from build123d import *

# Parameters (mm, degrees)
F0_W     = 40
F0_H     = 52
F1_DEPTH = 20
F2_D     = 7.5
F3_W     = 20
F3_H     = 52
F4_DEPTH = 50
F5_W     = 20
F5_H     = 52
F6_DEPTH = 50


with BuildPart() as f1:
    # F0 (on Front) → F1 (new body)
    with BuildSketch(Plane.XZ):
        Rectangle(F0_W, F0_H)
    extrude(amount=F1_DEPTH)

    # F2 (through all)
    with Locations(Plane(origin=(0, 0, 0), x_dir=(1, 0, 0), z_dir=(0, 1, 0))):
        with Locations((12, 20), (-12, 20), (12, -20), (-12, -20)):
            Hole(F2_D / 2)

    # F3 (on face) → F4 (join)
    with BuildSketch(Plane(origin=(-20, 0, 0), x_dir=(0, -1, 0), z_dir=(-1, 0, 0))):
        with Locations((10, 0)):
            Rectangle(F3_W, F3_H)
    extrude(amount=F4_DEPTH)

    # F5 (on face) → F6 (join)
    with BuildSketch(Plane.YZ.offset(20)):
        with Locations((-10, 0)):
            Rectangle(F5_W, F5_H)
    extrude(amount=F6_DEPTH)


solid = f1.part
Model file for the job. Use its own axes, mm. Give positions to 0.01 mm unless a question says otherwise; leave off trailing zeros. Loops run counter-clockwise (first coordinate to the right, second up) from the corner with the lowest first, then second, coordinate; pieces in that order, holes last.
Item 1: Slice it at C-C (x = -12). Write the cut outline in (y, z).
Check values:
outline: (-20, -26) - (0, -26) - (0, -23.75) - (-20, -23.75) - close; (-20, -16.25) - (0, -16.25) - (0, 16.25) - (-20, 16.25) - close; (-20, 23.75) - (0, 23.75) - (0, 26) - (-20, 26) - close
Item 2: Slice it at B-B (z = 20). Write the cut outline in (x, y), plus the area to 3 significant figures.
Check values:
outline: (-70, -20) - (-15.75, -20) - (-15.75, 0) - (-70, 0) - close; (-8.25, -20) - (8.25, -20) - (8.25, 0) - (-8.25, 0) - close; (15.75, -20) - (70, -20) - (70, 0) - (15.75, 0) - close
area: 2,500 mm2
Item 3: Drill centre lines: line 1 along X through (y, z) = (-7.25, 20); line 2 along Z through (x, y) = (12, -5.25); line 3 along X through (y, z) = (-5.75, 21). Where is each one in solid material? Low to high.
Check values:
line 1: x = -70 to -15.75, -8.25 to 8.25, 15.75 to 70
line 2: z = -26 to -23.75, -16.25 to 16.25, 23.75 to 26
line 3: x = -70 to -15.61, -8.39 to 8.39, 15.61 to 70
Item 4: Slice it at A-A (y = -12.25). Write the cut outline in (x, z), plus the area to 3 significant figures.
Check values:
outline: (-70, -26) - (70, -26) - (70, 26) - (-70, 26) - close; hole circle Ø7.5 at (-12, -20); hole circle Ø7.5 at (-12, 20); hole circle Ø7.5 at (12, -20); hole circle Ø7.5 at (12, 20)
area: 7,100 mm2
Item 5: Drop flat-ended pins along their axis: P1, Ø1, axis at x = 18.5, z = -4, coming from the +Y side; P2, Ø7, axis at x = 12, z = -20, coming from the -Y side. Give the stop position or say it passes through.
Check values:
P1: stops at y = 0
P2: passes through
Item 6: Mould opens along X. For faces 1 (the face through (-11.19, -10.14, 23.66)), 2 (the face through (-1, -10, 26)), 3 (the face through (70, -10, 0)), 4 (the face through (-70, -10, 0)) say: +X half, -X half, draft (parallel to the pull), parting line (faces both ways), or undercut.
Check values:
face 1: undercut
face 2: draft
face 3: +X half
face 4: -X half
